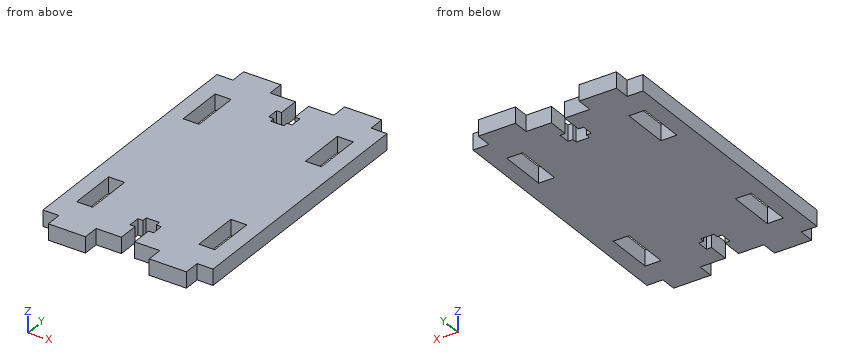
```python
from build123d import *

# Parameters (mm, degrees)
SKETCH_1_W          = 32
SKETCH_1_H          = 55
EXTRUDE_1_DEPTH     = 3
SKETCH_2_W          = 3
SKETCH_2_H          = 3
SKETCH_2_W_2        = 12
CUT_EXTRUDE_1_DEPTH = 4
SKETCH_3_W          = 3
SKETCH_3_H          = 9
CUT_EXTRUDE_2_DEPTH = 4
CUT_EXTRUDE_3_DEPTH = 10


with BuildPart() as part:
    # 스케치1 → 보스-돌출1 (new body)
    with BuildSketch(Plane.XY):
        with Locations((16, 27.5)):
            Rectangle(SKETCH_1_W, SKETCH_1_H)
    extrude(amount=EXTRUDE_1_DEPTH)

    # 스케치2 → 컷-돌출1 (cut, through all)
    with BuildSketch(Plane.XY.offset(3)):
        with Locations((1.5, 53.5)):
            Rectangle(SKETCH_2_W, SKETCH_2_H)
        with Locations((16, 53.5)):
            Rectangle(SKETCH_2_W_2, SKETCH_2_H)
        with Locations((30.5, 53.5)):
            Rectangle(SKETCH_2_W, SKETCH_2_H)
        with Locations((1.5, 1.5)):
            Rectangle(SKETCH_2_W, SKETCH_2_H)
        with Locations((16, 1.5)):
            Rectangle(SKETCH_2_W_2, SKETCH_2_H)
        with Locations((30.5, 1.5)):
            Rectangle(SKETCH_2_W, SKETCH_2_H)
    extrude(amount=-CUT_EXTRUDE_1_DEPTH, mode=Mode.SUBTRACT)

    # 스케치3 → 컷-돌출2 (cut, through all)
    with BuildSketch(Plane.XY.offset(3)):
        with Locations((4.5, 42.5)):
            Rectangle(SKETCH_3_W, SKETCH_3_H)
        with Locations((27.5, 42.5)):
            Rectangle(SKETCH_3_W, SKETCH_3_H)
        with Locations((27.5, 12.5)):
            Rectangle(SKETCH_3_W, SKETCH_3_H)
        with Locations((4.5, 12.5)):
            Rectangle(SKETCH_3_W, SKETCH_3_H)
    extrude(amount=-CUT_EXTRUDE_2_DEPTH, mode=Mode.SUBTRACT)

    # 스케치5 → 컷-돌출3 (cut)
    with BuildSketch(Plane.XY.offset(3)):
        Polygon((14.75, 10), (17.25, 10), (17.25, 9.08840284), (18.2, 9.08840284), (18.2, 6.88840284), (17.25, 6.88840284), (17.25, 3), (14.75, 3), (14.75, 6.88840284), (13.8, 6.88840284), (13.8, 9.08840284), (14.75, 9.08840284), align=None)
        Polygon((14.75, 45), (14.75, 45.91159716), (13.8, 45.91159716), (13.8, 48.11159716), (14.75, 48.11159716), (14.75, 52), (17.25, 52), (17.25, 48.11159716), (18.2, 48.11159716), (18.2, 45.91159716), (17.25, 45.91159716), (17.25, 45), align=None)
    extrude(amount=-CUT_EXTRUDE_3_DEPTH, mode=Mode.SUBTRACT)


solid = part.part
```
Model file for the job. Use its own axes, mm. Round coordinates to 2 decimals unless told otherwise and drop trailing zeros. Write each loop counter-clockwise with the first axis right and the second up, starting at its lowest first coordinate (ties: lowest second). Pieces come first, ordered by that corner, then holes. Notation, with made-up numbers: (-6.75, -36.75) -> (22.25, -36.75) arc R25 cw to (22.25, 2.25) -> close; hole circle Ø10 at (62.5, -36.5). An arc over 180 degrees is marked (long way). Answer as CSV lines item,"result".
1. Slice it at A-A, the plane y = 13. List the corners of the cut face in (x, z).
Resolved:
outline,"(0, 0) -> (3, 0) -> (3, 3) -> (0, 3) -> close; (6, 0) -> (26, 0) -> (26, 3) -> (6, 3) -> close; (29, 0) -> (32, 0) -> (32, 3) -> (29, 3) -> close"
2. Slice it at B-B, the plane x = 4.5. List the corners of the cut face in (y, z).
Resolved:
outline,"(0, 0) -> (8, 0) -> (8, 3) -> (0, 3) -> close; (17, 0) -> (38, 0) -> (38, 3) -> (17, 3) -> close; (47, 0) -> (55, 0) -> (55, 3) -> (47, 3) -> close"
3. Slice it at D-D, the plane x = 12. List the corners of the cut face in (y, z).
Resolved:
outline,"(3, 0) -> (52, 0) -> (52, 3) -> (3, 3) -> close"
4. Pin check, flat tips, straight feed: pin 1 Ø1.5 at (x, z) = (13.5, 1) entering from +Y; pin 2 Ø0.9 at (y, z) = (2, 1) entering from +X; pin 3 Ø1.5 at (x, z) = (12, 2) entering from -Y. Stop position of each tip, or through.
Resolved:
pin 1,"y = 52"
pin 2,"x = 29"
pin 3,"y = 3"
5. Slice it at C-C, the plane z = 2.4. State how many separate pieces and enclosed holes the cut face has, plus the area to 3 significant figures.
Resolved:
separate pieces,"1"
enclosed holes,"4"
area,"1,500 mm²"
6. Drill centre lines: line 1 (Y direction, x = 14.5, z = 2.65); line 2 (Y direction, x = 27, z = 2); line 3 (X direction, y = 44, z = 1.05). Where is each one in solid material? Low to high.
Resolved:
line 1,"3 to 6.89, 9.09 to 45.91, 48.11 to 52"
line 2,"0 to 8, 17 to 38, 47 to 55"
line 3,"0 to 3, 6 to 26, 29 to 32"
